from build123d import *

# Parameters (mm, degrees)
SKETCH1_R           = 1.75
BOSS_EXTRUDE1_DEPTH = 0.8
SKETCH2_W           = 20
SKETCH2_H           = 7.45
BOSS_EXTRUDE2_DEPTH = 5.2
SKETCH3_W           = 18
SKETCH3_H           = 4.5
CUT_EXTRUDE1_DEPTH  = 0.5
SKETCH4_R           = 0.65
BOSS_EXTRUDE3_DEPTH = 30


with BuildPart() as part:
    # Sketch1 → Boss-Extrude1 (new, symmetric)
    with BuildSketch(Plane(origin=(0, 0, 0), x_dir=(1, 0, 0), z_dir=(0, 1, 0))):
        with BuildLine():
            Line((29.5, -45), (-29.5, -45))
            ThreePointArc((-29.5, -45), (-30.914213562, -44.414213562), (-31.5, -43))
            Line((-31.5, -43), (-31.5, 43))
            ThreePointArc((-31.5, 43), (-30.914213562, 44.414213562), (-29.5, 45))
            Line((-29.5, 45), (29.5, 45))
            ThreePointArc((29.5, 45), (30.914213562, 44.414213562), (31.5, 43))
            Line((31.5, 43), (31.5, -43))
            ThreePointArc((31.5, -43), (30.914213562, -44.414213562), (29.5, -45))
        make_face()
        with Locations(Location((-28, 41.5, 0), (0, 0, 270))):
            Circle(SKETCH1_R, mode=Mode.SUBTRACT)
        with Locations(Location((28, 41.5, 0), (0, 0, 90))):
            Circle(SKETCH1_R, mode=Mode.SUBTRACT)
        with Locations(Location((28, -41.5, 0), (0, 0, 270))):
            Circle(SKETCH1_R, mode=Mode.SUBTRACT)
        with Locations(Location((-28, -41.5, 0), (0, 0, 90))):
            Circle(SKETCH1_R, mode=Mode.SUBTRACT)
    extrude(amount=BOSS_EXTRUDE1_DEPTH, both=True)

    # Sketch2 → Boss-Extrude2 (add)
    with BuildSketch(Plane(origin=(0, 0.8, 0), x_dir=(1, 0, 0), z_dir=(0, 1, 0))):
        with Locations((0, -41.275)):
            Rectangle(SKETCH2_W, SKETCH2_H)
    extrude(amount=BOSS_EXTRUDE2_DEPTH)

    # Sketch3 → Cut-Extrude1 (cut)
    with BuildSketch(Plane.XY.offset(45)):
        with Locations((0, 3.4)):
            Rectangle(SKETCH3_W, SKETCH3_H)
    extrude(amount=-CUT_EXTRUDE1_DEPTH, mode=Mode.SUBTRACT)

    # Sketch4 → Boss-Extrude3 (add)
    with BuildSketch(Plane.XY.offset(44.5)):
        with Locations((-8, 3.4)):
            Circle(SKETCH4_R)
        with Locations((-5.75, 3.4)):
            Circle(SKETCH4_R)
        with Locations((-3.5, 3.4)):
            Circle(SKETCH4_R)
        with Locations((-1.25, 3.4)):
            Circle(SKETCH4_R)
        with Locations((1, 3.4)):
            Circle(SKETCH4_R)
        with Locations((3.25, 3.4)):
            Circle(SKETCH4_R)
        with Locations((5.5, 3.4)):
            Circle(SKETCH4_R)
        with Locations((7.75, 3.4)):
            Circle(SKETCH4_R)
    extrude(amount=BOSS_EXTRUDE3_DEPTH)


solid = part.part
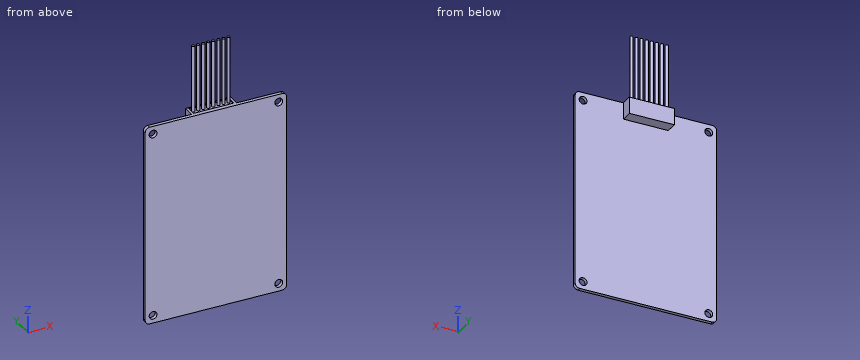
Could you check a few things on this model? Use its own coordinates, in mm. Give positions to 0.01 mm unless a question says otherwise; leave off trailing zeros. Write each loop counter-clockwise with the first axis right and the second up, starting at its lowest first coordinate (ties: lowest second). Pieces come first, ordered by that corner, then holes. Notation, with made-up numbers: (-9.5, 16.5) - (15.5, 16.5) arc R16 ccw to (15.5, 34.5) - close; hole circle Ø7 at (30, 62). An arc over 180 degrees is marked (long way). Use CSV: the item, a comma, the result in double quotes. Start each with the question number.
Item 1: I want a section at B-B, the plane x = 21.5. Please give me the cut outline in (y, z).
Item 2: If I drill on line 1 along X through (y, z) = (0.1, -41.5); line 2 along Y through (x, z) = (12, -32); line 3 along Z through (x, y) = (-26.5, 0.5), over which ranges is the centre line in solid material (lowest first)?
Item 3: I want a section at A-A, the plane z = -41.5. Please give me the cut outline in (x, y), then the cut area to 3 significant figures.
Item 4: I'm going to push flat-ended pins straight in: pin 1 (2 mm diameter, centred on x = -28, z = 41.5, fed in from +Y); pin 2 (12 mm diameter, centred on x = -23.5, z = -7, fed in from +Y); pin 3 (1.6 mm diameter, centred on y = 3, z = 41, fed in from +X). Where does each tip first touch, or does it pass through?
Item 5: I want a section at C-C, the plane z = 31.5. Please give me the cut outline in (x, y).
Findings:
1,outline,"(-0.8, -45) - (0.8, -45) - (0.8, 45) - (-0.8, 45) - close"
2,line 1,"x = -31.5 to -29.75, -26.25 to 26.25, 29.75 to 31.5"
2,line 2,"y = -0.8 to 0.8"
2,line 3,"z = -45 to -42.4, -40.6 to 40.6, 42.4 to 45"
3,outline,"(-31.5, -0.8) - (-29.75, -0.8) - (-29.75, 0.8) - (-31.5, 0.8) - close; (-26.25, -0.8) - (26.25, -0.8) - (26.25, 0.8) - (-26.25, 0.8) - close; (29.75, -0.8) - (31.5, -0.8) - (31.5, 0.8) - (29.75, 0.8) - close"
3,area,"89.6 mm2"
4,pin 1,"passes through"
4,pin 2,"stops at y = 0.8"
4,pin 3,"stops at x = 10"
5,outline,"(-31.5, -0.8) - (31.5, -0.8) - (31.5, 0.8) - (-31.5, 0.8) - close"
